from build123d import *

# Parameters (mm, degrees)
SKETCH1_W           = 143.51
SKETCH1_H           = 71.12
BOSS_EXTRUDE1_DEPTH = 3.81
SKETCH2_W           = 7.62
SKETCH2_H           = 2.54
BOSS_EXTRUDE3_DEPTH = 8.89
SKETCH5_R           = 2
CUT_EXTRUDE2_DEPTH  = 90.125877794


with BuildPart() as part:
    # Sketch1 → Boss-Extrude1 (new body)
    with BuildSketch(Plane(origin=(0, 0, 0), x_dir=(1, 0, 0), z_dir=(0, 1, 0))):
        with Locations((-3.577228739, -9.256847507)):
            Rectangle(SKETCH1_W, SKETCH1_H)
    extrude(amount=BOSS_EXTRUDE1_DEPTH)

    # Sketch2 → Boss-Extrude3 (add)
    with BuildSketch(Plane(origin=(0, 3.81, 0), x_dir=(1, 0, 0), z_dir=(0, 1, 0))):
        with Locations((-46.122228739, 27.573152493)):
            Rectangle(SKETCH2_W, SKETCH2_H)
        with Locations((38.967771261, 27.573152493)):
            Rectangle(SKETCH2_W, SKETCH2_H)
        with Locations((-49.932228739, -46.086847507)):
            Rectangle(SKETCH2_W, SKETCH2_H)
        with Locations((38.967771261, -46.086847507)):
            Rectangle(SKETCH2_W, SKETCH2_H)
    extrude(amount=-BOSS_EXTRUDE3_DEPTH)

    # Sketch5 → Cut-Extrude2 (cut, through all)
    with BuildSketch(Plane(origin=(0, 0, 0), x_dir=(-1, 0, 0), z_dir=(0, -1, 0))):
        with Locations(Location((-46.587771261, -27.036847507, 0), (0, 0, 90))):
            Circle(SKETCH5_R)
        with Locations(Location((-46.587771261, 0.903152493, 0), (0, 0, 90))):
            Circle(SKETCH5_R)
    extrude(amount=-CUT_EXTRUDE2_DEPTH, mode=Mode.SUBTRACT)


solid = part.part
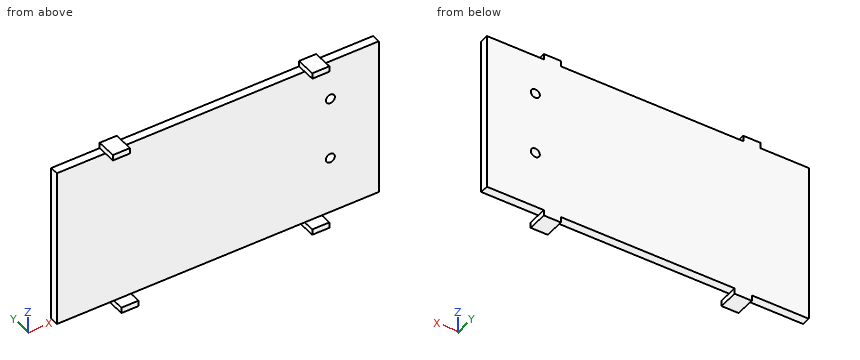
Model file for the job. Use its own axes, mm. Give positions to 0.01 mm unless a question says otherwise; leave off trailing zeros. Loops run counter-clockwise (first coordinate to the right, second up) from the corner with the lowest first, then second, coordinate; pieces in that order, holes last.
1) Wall check: line 1 (Z direction, x = -47.5, y = -4.25); line 2 (Y direction, x = -32.5, z = -22); line 3 (Z direction, x = 7, y = 0.25). Give the ranges that are in metal, low to high.
2) Flat gauge pins, fed straight in: pin 1 Ø12 at (x, z) = (53, 32.5) entering from -Y; pin 2 Ø4 at (x, y) = (-68.5, 1.5) entering from -Z; pin 3 Ø3 at (y, z) = (1, 46.5) entering from +X; pin 4 Ø5 at (x, z) = (46.59, 27.04) entering from +Y. Where does each tip first touch, or does it go through?
3) Saw through at A-A (y = -3.5). Write the cut outline in (x, z).
4) Saw through at C-C (z = 21). Write the cut outline in (x, y), plus the area to 3 significant figures.
5) Saw through at B-B (x = -48). Write the cut outline in (y, z).
Answer block:
1. line 1: z = -28.84 to -26.3, 44.82 to 47.36
1. line 2: y = 0 to 3.81
1. line 3: z = -26.3 to 44.82
2. pin 1: stops at y = 0
2. pin 2: stops at z = -26.3
2. pin 3: stops at x = 42.78
2. pin 4: stops at y = 3.81
3. outline: (-53.74, 44.82) - (-46.12, 44.82) - (-46.12, 47.36) - (-53.74, 47.36) - close; (-49.93, -28.84) - (-42.31, -28.84) - (-42.31, -26.3) - (-49.93, -26.3) - close; (35.16, -28.84) - (42.78, -28.84) - (42.78, -26.3) - (35.16, -26.3) - close; (35.16, 44.82) - (42.78, 44.82) - (42.78, 47.36) - (35.16, 47.36) - close
4. outline: (-75.33, 0) - (68.18, 0) - (68.18, 3.81) - (-75.33, 3.81) - close
4. area: 547 mm2
5. outline: (-5.08, -28.84) - (3.81, -28.84) - (3.81, 47.36) - (-5.08, 47.36) - (-5.08, 44.82) - (0, 44.82) - (0, -26.3) - (-5.08, -26.3) - close
